from build123d import *

# Parameters (mm, degrees)
SKETCH1_R           = 1.55
BOSS_EXTRUDE1_DEPTH = 3.175
CUT_EXTRUDE1_DEPTH  = 4.175
FILLET1_R           = 8.89
SKETCH3_R           = 1.5
CUT_EXTRUDE2_DEPTH  = 4.175
SKETCH4_R           = 0.9525
CUT_EXTRUDE3_DEPTH  = 4.175
FILLET2_R           = 6.35


with BuildPart() as part:
    # Sketch1 → Boss-Extrude1 (new body)
    with BuildSketch(Plane(origin=(0, 0, 0), x_dir=(0, 0, -1), z_dir=(1, 0, 0))):
        with BuildLine():
            Line((69.85, 75.565), (-82.55, 75.565))
            Line((-82.55, 75.565), (-82.55, -75.565))
            Line((-82.55, -75.565), (69.85, -75.565))
            ThreePointArc((69.85, -75.565), (78.830256121, -71.845256121), (82.55, -62.865))
            Line((82.55, -62.865), (82.55, 62.865))
            ThreePointArc((82.55, 62.865), (78.830256121, 71.845256121), (69.85, 75.565))
        make_face()
        with Locations((69.85, 62.865)):
            Circle(SKETCH1_R, mode=Mode.SUBTRACT)
    extrude(amount=BOSS_EXTRUDE1_DEPTH)

    # Sketch2 → Cut-Extrude1 (cut, through all)
    with BuildSketch(Plane(origin=(3.175, 0, 0), x_dir=(0, 0, -1), z_dir=(1, 0, 0))):
        with BuildLine():
            Line((-63.5, -10.915332745), (-63.5, -75.565))
            Line((-63.5, -75.565), (-50.8, -75.565))
            ThreePointArc((-50.8, -75.565), (-54.005053677, -42.622362446), (-63.5, -10.915332745))
        make_face()
        with BuildLine():
            Line((-82.55, 75.565), (-82.55, 62.865))
            ThreePointArc((-82.55, 62.865), (-82.417420191, 69.220528969), (-82.019911437, 75.565))
            Line((-82.019911437, 75.565), (-82.55, 75.565))
        make_face()
        with BuildLine():
            Line((-82.55, -75.565), (-63.5, -75.565))
            Line((-63.5, -75.565), (-63.5, -10.915332745))
            ThreePointArc((-63.5, -10.915332745), (-77.710665491, 24.765), (-82.55, 62.865))
            Line((-82.55, 62.865), (-82.55, -75.565))
        make_face()
    extrude(amount=-CUT_EXTRUDE1_DEPTH, mode=Mode.SUBTRACT)

    # Fillet1
    fillet1_edges = [part.edges().sort_by_distance(p)[0] for p in [
        (1.5875, 75.565, 82.019911437),
    ]]
    fillet(fillet1_edges, radius=FILLET1_R)

    # Sketch3 → Cut-Extrude2 (cut, through all)
    with BuildSketch(Plane(origin=(3.175, 0, 0), x_dir=(0, 0, -1), z_dir=(1, 0, 0))):
        with Locations((-60.325, 62.865)):
            Circle(SKETCH3_R)
    extrude(amount=-CUT_EXTRUDE2_DEPTH, mode=Mode.SUBTRACT)

    # Sketch4 → Cut-Extrude3 (cut, through all)
    with BuildSketch(Plane(origin=(3.175, 0, 0), x_dir=(0, 0, -1), z_dir=(1, 0, 0))):
        with Locations((-74.561915864, 73.9775)):
            Circle(SKETCH4_R)
        with Locations((-62.57206458, -9.313350112)):
            Circle(SKETCH4_R)
    extrude(amount=-CUT_EXTRUDE3_DEPTH, mode=Mode.SUBTRACT)

    # Fillet2
    fillet2_edges = [part.edges().sort_by_distance(p)[0] for p in [
        (1.5875, -75.565, 50.8),
    ]]
    fillet(fillet2_edges, radius=FILLET2_R)


solid = part.part
Design review of the part built by this model. Coordinates are the model's own, in mm. Round coordinates to 2 decimals unless told otherwise and drop trailing zeros. Loops run counter-clockwise (first coordinate to the right, second up) from the corner with the lowest first, then second, coordinate; pieces in that order, holes last. Notation, with made-up numbers: M 65.5,48.5 L 120.5,48.5 A25 cw 120.5,79.5 Z; hole C 31,35 d1. An arc over 180 degrees is marked long. Answer as a JSON object with one key per item and string values.
Item 1: We need section C-C on z = 66. Give the boundary of the cut face in (x, y) (3 decimals).
Answer sheet:
{"outline": "M 0,-6.204 L 3.175,-6.204 L 3.175,75.565 L 0,75.565 Z"}
Item 2: We need section A-A on x = 2.3. State how many separate pieces and enclosed holes the cut face has, and give its area (3 significant figures).
Answer sheet:
{"separate pieces": "1", "enclosed holes": "4", "area": "22,600 mm^2"}
Item 3: Wall thickness on L1, parallel to Y at x = 2.2, z = -69.85 (3 decimals); L2, parallel to Z at x = 1.95, y = -50.5; L3, parallel to Z at x = 2.95, y = 30.5: over which ranges is each line inside the solid? List them lowest first. Write a range as from..to.
Answer sheet:
{"L1": "y = -75.565..61.315, 64.415..75.565", "L2": "z = -82.55..52.65", "L3": "z = -82.55..79.07"}
Item 4: We need section B-B on y = 10. Give the boundary of the cut face in (x, z) (3 decimals), and give its area (3 significant figures).
Answer sheet:
{"outline": "M 0,-82.55 L 3.175,-82.55 L 3.175,73.087 L 0,73.087 Z", "area": "494 mm^2"}
